from build123d import *

# Parameters (mm, degrees)
SKETCH1_W           = 13.824903871
SKETCH1_H           = 8.964949161
BOSS_EXTRUDE1_DEPTH = 5
SKETCH2_W           = 13.088608924
SKETCH2_H           = 8.309427022
CUT_EXTRUDE1_DEPTH  = 4.8
BOSS_EXTRUDE2_DEPTH = 1.8
SKETCH4_R           = 1.4
CUT_EXTRUDE3_DEPTH  = 1.8
SKETCH7_W           = 0.440803266
SKETCH7_H           = 2.270686526
CUT_EXTRUDE4_DEPTH  = 18.162117599
SKETCH9_W           = 3.10665333
SKETCH9_H           = 3.017419
BOSS_EXTRUDE3_DEPTH = 17
SKETCH11_W          = 3.315667702
SKETCH11_H          = 0.539606784
CUT_EXTRUDE11_DEPTH = 1


with BuildPart() as part:
    # Sketch1 → Boss-Extrude1 (new body)
    with BuildSketch(Plane(origin=(0, 0, 0), x_dir=(1, 0, 0), z_dir=(0, 1, 0))):
        with Locations((6.912451936, -4.48247458)):
            Rectangle(SKETCH1_W, SKETCH1_H)
    extrude(amount=BOSS_EXTRUDE1_DEPTH)

    # Sketch2 → Cut-Extrude1 (cut)
    with BuildSketch(Plane(origin=(0, 5, 0), x_dir=(1, 0, 0), z_dir=(0, 1, 0))):
        with Locations((6.945565783, -4.53797661)):
            Rectangle(SKETCH2_W, SKETCH2_H)
    extrude(amount=-CUT_EXTRUDE1_DEPTH, mode=Mode.SUBTRACT)

    # Sketch3 → Boss-Extrude2 (add)
    with BuildSketch(Plane(origin=(0, 0.2, 0), x_dir=(1, 0, 0), z_dir=(0, 1, 0))):
        Polygon((8.401261321, -0.383263099), (8.201261321, -0.383263099), (8.201261321, -4.183263099), (0.401261321, -4.183263099), (0.401261321, -4.383263099), (8.401261321, -4.383263099), align=None)
    extrude(amount=BOSS_EXTRUDE2_DEPTH)

    # Sketch4 → Cut-Extrude3 (cut)
    with BuildSketch(Plane.ZY):
        with Locations((6.651943346, 1.742318178)):
            Circle(SKETCH4_R)
    extrude(amount=-CUT_EXTRUDE3_DEPTH, mode=Mode.SUBTRACT)

    # Sketch7 → Cut-Extrude4 (cut, through all)
    with BuildSketch(Plane(origin=(0, 0.2, 0), x_dir=(1, 0, 0), z_dir=(0, 1, 0))):
        with Locations((12.838352813, -7.176919556)):
            Rectangle(SKETCH7_W, SKETCH7_H)
    extrude(amount=-CUT_EXTRUDE4_DEPTH, mode=Mode.SUBTRACT)

    # Sketch9 → Boss-Extrude3 (add)
    with BuildSketch(Plane(origin=(0, 5, 0), x_dir=(1, 0, 0), z_dir=(0, 1, 0))):
        Polygon((13.489870245, -4.115580834), (10.0509272, -4.115580834), (10.0509272, -0.383263099), (10.0509272, 0), (13.824903871, 0), (13.824903871, -4.115580834), align=None)
        with Locations((11.93654358, -2.24927503)):
            Rectangle(SKETCH9_W, SKETCH9_H, mode=Mode.SUBTRACT)
    extrude(amount=BOSS_EXTRUDE3_DEPTH)

    # Sketch11 → Cut-Extrude11 (cut)
    with BuildSketch(Plane(origin=(0, 0, 0), x_dir=(-1, 0, 0), z_dir=(0, 0, -1))):
        with Locations((-11.708761051, 4.669803392)):
            Rectangle(SKETCH11_W, SKETCH11_H)
    extrude(amount=-CUT_EXTRUDE11_DEPTH, mode=Mode.SUBTRACT)


solid = part.part
Can you work these out from the model? Positions are in its coordinate system, mm. A direction names the side the tool comes from. Give positions to 0.01 mm unless a question says otherwise; leave off trailing zeros. Order: outer loops, then holes, each group sorted by start corner. A loop starts at its lowest first (then second) coordinate and runs counter-clockwise, first axis right, second up. Notation, with made-up numbers: M -28.75,-23.5 L 21.25,-23.5 A24 ccw 21.25,11.5 Z; hole C 58.25,76 d11. An arc over 180 degrees is marked long. One line per question, with ' | ' between items.
Item 1: For faces 1 (the face through (12, 13, 3.758)), 2 (the face through (10.051, 13, 2)), 3 (the face through (12, 22, 0.2)), 4 (the face through (12, 13, 4.116)), which set-ups out of +Z, -Z, +X, -X, +Y, -Y let a thin tool reach every point of the face, with its end or its side?
Answer block:
face 1: +Y | face 2: +Z, -Z, -X, +Y | face 3: +Z, -Z, +X, -X, +Y | face 4: +Z, +X, -X, +Y
Item 2: Please list where these lines run through material, in increasing order: L1, parallel to X at y = 17, z = 2.5; L2, parallel to Z at x = 2.5, y = 3.75; L3, parallel to Y at x = 4.25, z = 5.25.
Answer block:
L1: x = 10.05 to 10.38, 13.49 to 13.82 | L2: z = 0 to 0.38, 8.69 to 8.96 | L3: y = 0 to 0.2
Item 3: Suppose I cut it at D-D, the plane z = 2. Write out the boundary of the cut face in (x, y), then the cut area to 3 significant figures.
Answer block:
outline: M 0,0 L 13.82,0 L 13.82,22 L 13.49,22 L 13.49,0.2 L 8.4,0.2 L 8.4,2 L 8.2,2 L 8.2,0.2 L 0.4,0.2 L 0.4,5 L 0,5 Z; M 10.05,5 L 10.38,5 L 10.38,22 L 10.05,22 Z | area: 18.0 mm2
Item 4: Suppose I cut it at A-A, the plane x = 12. Write out the boundary of the cut face in (y, z).
Answer block:
outline: M 0,0 L 4.4,0 L 4.4,0.38 L 0.2,0.38 L 0.2,8.69 L 5,8.69 L 5,8.96 L 0,8.96 Z; M 4.94,0 L 22,0 L 22,0.74 L 5,0.74 L 5,0.38 L 4.94,0.38 Z; M 5,3.76 L 22,3.76 L 22,4.12 L 5,4.12 Z
Item 5: I'm going to push flat-ended pins straight in: pin 1 Ø2.5 at (x, y) = (11, 17.5) entering from +Z; pin 2 Ø1.5 at (x, z) = (11, 6.5) entering from +Y; pin 3 Ø8 at (x, y) = (5.5, 7) entering from -Z; pin 4 Ø2.5 at (x, z) = (7.5, 4) entering from +Y. Where does each tip first touch, or does it pass through?
Answer block:
pin 1: stops at z = 4.12 | pin 2: stops at y = 0.2 | pin 3: stops at z = 0 | pin 4: stops at y = 2
Item 6: We'd pull the mould along Y, two halves only. Please class faces 5 (the face through (8.201, 1, 2)), 6 (the face through (4, 0.2, 2)), 7 (the face through (0.198, 1.206, 7.945)), 8 (the face through (7, 3, 0.383)): released by +Y, released by -Y, zero draft, split by the parting line, or undercut.
Answer block:
face 5: zero draft | face 6: released by +Y | face 7: undercut | face 8: undercut
Item 7: Suppose I cut it at B-B, the plane z = 6.5. Write out the boundary of the cut face in (x, y).
Answer block:
outline: M 0,0 L 12.62,0 L 12.62,0.2 L 0.4,0.2 L 0.4,0.35 L 0,0.35 Z; M 0,3.13 L 0.4,3.13 L 0.4,5 L 0,5 Z; M 13.06,0 L 13.82,0 L 13.82,5 L 13.49,5 L 13.49,0.2 L 13.06,0.2 Z
Item 8: Suppose I cut it at C-C, the plane y = 5.25. Write out the boundary of the cut face in (x, z).
Answer block:
outline: M 10.05,0 L 13.82,0 L 13.82,4.12 L 10.05,4.12 Z; hole M 10.38,0.74 L 13.49,0.74 L 13.49,3.76 L 10.38,3.76 Z
